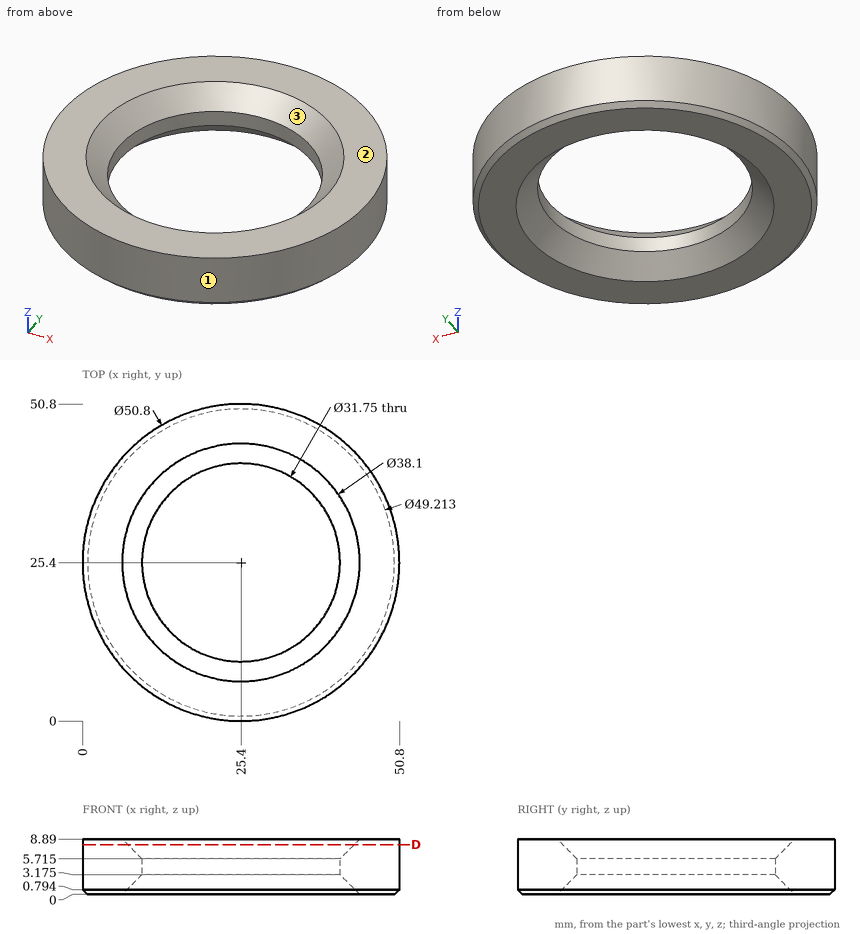
Drawing for the job (mm, zero at the part's lowest x, y, z). Give positions to 0.01 mm unless a question says otherwise; leave off trailing zeros. Write each loop counter-clockwise with the first axis right and the second up, starting at its lowest first coordinate (ties: lowest second). Pieces come first, ordered by that corner, then holes. Notation, with made-up numbers: (44, 49) -> (67, 49) arc R12 ccw to (67, 65) -> close; hole circle Ø1 at (-33.75, 24). An arc over 180 degrees is marked (long way). Put each result on its own line as item: value. Start each with the question number.
Item 1: Cut at D-D (z = 8). List the corners of the cut face in (x, y).
Item 2: Pin check, flat tips, straight feed: pin 1 Ø1.5 at (y, z) = (18.5, 4.5) entering from +X; pin 2 Ø4 at (x, y) = (19.5, 11.5) entering from +Z; pin 3 Ø8 at (x, y) = (36.5, 10) entering from +Z; pin 4 Ø2 at (x, z) = (33, 7) entering from +Y. Stop position of each tip, or through.
Item 3: Pull direction Y, two halves, no side cores. Call the marked faces 1, 2 and 3: pulls with the +Y half, pulls with the -Y half, needs draft (parallel to the pull), parting line crosses it, or undercut.
Item 4: Wall check: L1, parallel to Y at x = 25.4, z = 4.3 (1 decimal); L2, parallel to X at y = 35, z = 2.25 (1 decimal); L3, parallel to X at y = 26.5, z = 6 (1 decimal). Give the ranges that are in metal, low to high. Write a range as [from, to].
Answer list:
1. outline: circle Ø50.8 at (25.4, 25.4); hole circle Ø36.32 at (25.4, 25.4)
2. pin 1: stops at x = 50.04
2. pin 2: stops at z = 6.94
2. pin 3: stops at z = 8.89
2. pin 4: stops at y = 49.93
3. face 1: parting line crosses it
3. face 2: needs draft
3. face 3: undercut
4. L1: y = [0, 9.5], [41.3, 50.8]
4. L2: x = [1.9, 11.6], [39.2, 48.9]
4. L3: x = [0, 9.3], [41.5, 50.8]
